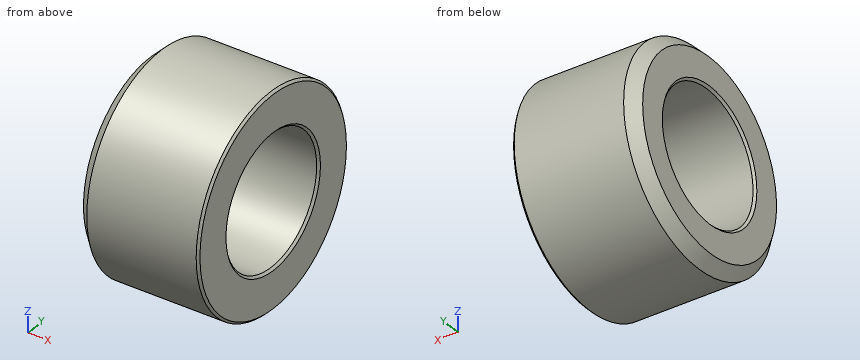
from build123d import *

# Parameters (mm, degrees)
ESQUISSE1_W     = 5.5
ESQUISSE1_H     = 1.85
CHANFREIN1_SIZE = 0.1
CHANFREIN2_SIZE = 0.5


with BuildPart() as part:
    # Esquisse1 → Révolution1 (revolve)
    with BuildSketch(Plane.XY):
        with Locations((0, 3.825)):
            Rectangle(ESQUISSE1_W, ESQUISSE1_H)
    revolve(axis=Axis((0, 0, 0), (-1, 0, 0)))

    # Chanfrein1
    chanfrein1_edges = [part.edges().sort_by_distance(p)[0] for p in [
        (2.75, -2.9, 0),
        (-2.75, -2.9, 0),
        (2.75, -4.75, 0),
    ]]
    chamfer(chanfrein1_edges, length=CHANFREIN1_SIZE)

    # Chanfrein2
    chanfrein2_edges = [part.edges().sort_by_distance(p)[0] for p in [
        (-2.75, -4.75, 0),
    ]]
    chamfer(chanfrein2_edges, length=CHANFREIN2_SIZE)


solid = part.part
Read the model definition and answer for the solid it produces. Units are mm, in the model's axes. Give positions to 0.01 mm unless a question says otherwise; leave off trailing zeros. Loops run counter-clockwise (first coordinate to the right, second up) from the corner with the lowest first, then second, coordinate; pieces in that order, holes last. Notation, with made-up numbers: (24, 41) -> (68, 41) arc R37 cw to (68, 79) -> close; hole circle Ø10 at (51, 60). An arc over 180 degrees is marked (long way). Answer as CSV lines item,"result".
Item 1: Each of these flat-tipped pins is pushed along its axis until it touches: pin 1 (3 mm diameter, centred on x = 2, y = 2, fed in from -Z); pin 2 (1 mm diameter, centred on x = -0.5, y = -3, fed in from +Z). Where does it stop, or does it pass through?
Returned:
pin 1,"stops at z = -4.72"
pin 2,"stops at z = 4.04"
Item 2: Consider line 1 (Z direction, x = -1.3, y = 0); line 2 (Z direction, x = 0.2, y = -1.5). Determine where each line is inside the solid, lowest interval first. Write a range as [from, to].
Returned:
line 1,"z = [-4.75, -2.9], [2.9, 4.75]"
line 2,"z = [-4.51, -2.48], [2.48, 4.51]"
Item 3: Find section A-A on y = 0. Give the vertices of the cut face in (x, z), plus the area to 3 significant figures.
Returned:
outline,"(-2.75, -4.25) -> (-2.25, -4.75) -> (2.65, -4.75) -> (2.75, -4.65) -> (2.75, -3) -> (2.65, -2.9) -> (-2.65, -2.9) -> (-2.75, -3) -> close; (-2.75, 3) -> (-2.65, 2.9) -> (2.65, 2.9) -> (2.75, 3) -> (2.75, 4.65) -> (2.65, 4.75) -> (-2.25, 4.75) -> (-2.75, 4.25) -> close"
area,"20.1 mm²"
Item 4: Find section C-C on x = -2.4. Give the vertices of the cut face in (y, z).
Returned:
outline,"circle Ø9.2 at (0, 0); hole circle Ø5.8 at (0, 0)"
Item 5: Find section D-D on x = 2.35. Give the vertices of the cut face in (y, z).
Returned:
outline,"circle Ø9.5 at (0, 0); hole circle Ø5.8 at (0, 0)"
